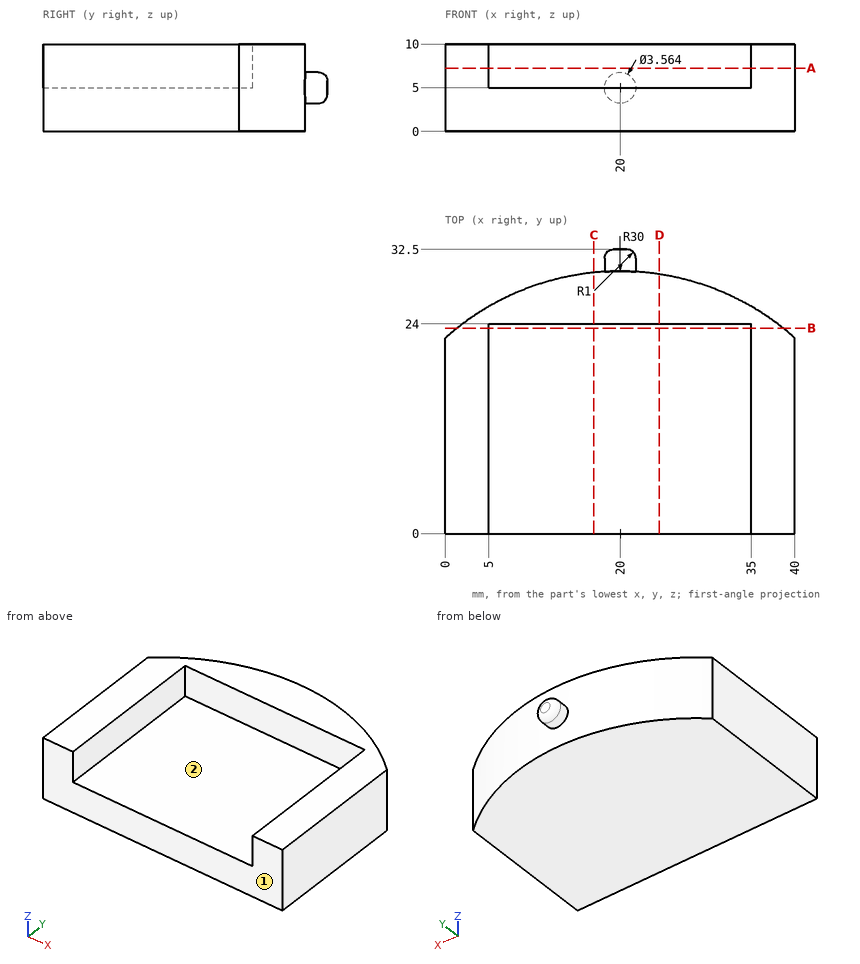
Could you check a few things on this drawing? It's one solid part, dimensions in mm from its lowest x, y, z. A direction names the side the tool comes from. Round coordinates to 2 decimals unless told otherwise and drop trailing zeros. Order: outer loops, then holes, each group sorted by start corner. A loop starts at its lowest first (then second) coordinate and runs counter-clockwise, first axis right, second up.
Q1. Imagine slicing it at D-D, the plane x = 24.5. List the corners of the cut face in (y, z) for me.
Geometry says:
outline: (0, 0) - (29.66, 0) - (29.66, 10) - (24, 10) - (24, 5) - (0, 5) - close
Q2. Which directions (+Z, -Z, +X, -X, +Y, -Y) give clear straight access to the entire face, cutting with the end or side of a thin tool? Please do the marked faces 1 and 2.
Geometry says:
face 1: +Z, -Z, +X, -X, -Y
face 2: +Z, -Y
Q3. Imagine slicing it at B-B, the plane y = 23.5. List the corners of the cut face in (x, z) for me.
Geometry says:
outline: (1.35, 0) - (38.65, 0) - (38.65, 10) - (35, 10) - (35, 5) - (5, 5) - (5, 10) - (1.35, 10) - close
Q4. Imagine slicing it at A-A, the plane z = 7.25. List the corners of the cut face in (x, y) for me, then the cut area to 3 significant figures.
Geometry says:
outline: (0, 0) - (5, 0) - (5, 24) - (35, 24) - (35, 0) - (40, 0) - (40, 22.36) arc R30 ccw to (0, 22.36) - close
area: 384 mm2
Q5. I'm going to push flat-ended pins straight in: P1, Ø12, axis at x = 28.5, y = 21, coming from the +Z side; P2, Ø2, axis at x = 16, z = 8, coming from the +Y side; P3, Ø4, axis at y = 29, z = 4.5, coming from the +X side; P4, Ø7, axis at x = 13, y = 10.5, coming from the +Z side. Where does each tip first touch, or does it pass through?
Geometry says:
P1: stops at z = 10
P2: stops at y = 29.85
P3: stops at x = 33.08
P4: stops at z = 5
Q6. Please list where these lines run through material, in increasing order: probe 1 along X at (y, z) = (17, 8); probe 2 along Z at (x, y) = (22, 19.5); probe 3 along Y at (x, z) = (19.5, 2).
Geometry says:
probe 1: x = 0 to 5, 35 to 40
probe 2: z = 0 to 5
probe 3: y = 0 to 30
Q7. Imagine slicing it at C-C, the plane x = 17. List the corners of the cut face in (y, z) for me, then the cut area to 4 significant figures.
Geometry says:
outline: (0, 0) - (29.85, 0) - (29.85, 10) - (24, 10) - (24, 5) - (0, 5) - close
area: 178.5 mm2
